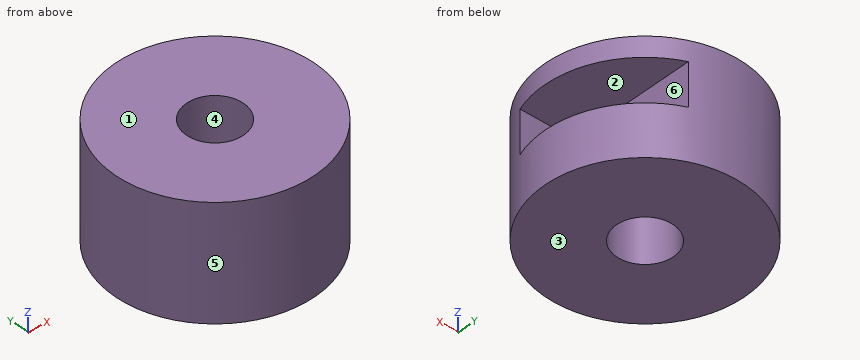
```python
from build123d import *

# Parameters (mm, degrees)
BOX_W             = 30
BOX_H             = 30
BOX_DEPTH         = 7.5
CYLINDER001_R     = 5
CYLINDER001_DEPTH = 40
CYLINDER_R        = 17.5
CYLINDER_DEPTH    = 20


with BuildPart() as cube:
    # Box → Box (new body)
    with BuildSketch(Plane(origin=(7, -6, 9), x_dir=(1, 0, 0), z_dir=(0, 0, 1))):
        with Locations((15, 15)):
            Rectangle(BOX_W, BOX_H)
    extrude(amount=BOX_DEPTH)


with BuildPart() as cylinder001:
    # Cylinder001 → Cylinder001 (new body)
    with BuildSketch(Plane.XY.offset(-10)):
        Circle(CYLINDER001_R)
    extrude(amount=CYLINDER001_DEPTH)


with BuildPart() as mount_bottom:
    # Cylinder → Cylinder (new body)
    with BuildSketch(Plane.XY):
        Circle(CYLINDER_R)
    extrude(amount=CYLINDER_DEPTH)

    # Cut: cut Cylinder001
    add(cylinder001.part, mode=Mode.SUBTRACT)

    # Cut001: cut Cube
    add(cube.part, mode=Mode.SUBTRACT)


solid = mount_bottom.part
```
The listing builds one solid part. Answer for the finished solid, in the listing's coordinates (mm). Face numbers are marked on the shaded views. A direction names the side the tool comes from. Give positions to 0.01 mm unless a question says otherwise; leave off trailing zeros. Order: outer loops, then holes, each group sorted by start corner. A loop starts at its lowest first (then second) coordinate and runs counter-clockwise, first axis right, second up. Notation, with made-up numbers: (80, 32.25) -> (134, 32.25) arc R7 ccw to (134, 44.25) -> close; hole circle Ø11 at (88.5, 77.25). An arc over 180 degrees is marked (long way). One line per item, written item: value.
1) Determine the mould class of the marked faces 3, 4, 5 and 6 for opening direction X: pulls with the +X half, pulls with the -X half, needs draft (parallel to the pull), parting line crosses it, or undercut.
Reported:
face 3: needs draft
face 4: undercut
face 5: parting line crosses it
face 6: pulls with the +X half
2) Find the intervals of material crossed by line 1 (Z direction, x = 15, y = 7); line 2 (Y direction, x = 0, z = 12); line 3 (X direction, y = 3.5, z = 7), in increasing order.
Reported:
line 1: z = 0 to 9, 16.5 to 20
line 2: y = -17.5 to -5, 5 to 17.5
line 3: x = -17.15 to -3.57, 3.57 to 17.15
3) Flat-ended cylindrical pins translate along their axes: P1, Ø1.5, axis at x = -10, z = 13, coming from the -Y side; P2, Ø6, axis at y = 10.5, z = 2.5, coming from the -X side; P3, Ø10, axis at y = 7, z = 7, coming from the +X side; P4, Ø8, axis at y = 3.5, z = 16.5, coming from the +X side. Find the tip coordinate at first contact, or state that the pin passes through.
Reported:
P1: stops at y = -14.86
P2: stops at x = -15.81
P3: stops at x = 17.39
P4: stops at x = 17.5
4) Find section A-A, the plane y = 0. Determine the outline of the cut face in (x, z), plus the area to 3 significant figures.
Reported:
outline: (-17.5, 0) -> (-5, 0) -> (-5, 20) -> (-17.5, 20) -> close; (5, 0) -> (17.5, 0) -> (17.5, 9) -> (7, 9) -> (7, 16.5) -> (17.5, 16.5) -> (17.5, 20) -> (5, 20) -> close
area: 421 mm^2
5) Find section B-B, the plane x = 0. Determine the outline of the cut face in (y, z).
Reported:
outline: (-17.5, 0) -> (-5, 0) -> (-5, 20) -> (-17.5, 20) -> close; (5, 0) -> (17.5, 0) -> (17.5, 20) -> (5, 20) -> close
6) A tool of negligible diameter and unlimited length cuts with its end or side. For the marked faces 1 and 2, from which of +Z, -Z, +X, -X, +Y, -Y can it reach the whole face along a straight path? Write none if from no direction.
Reported:
face 1: +Z, +X, -X, +Y, -Y
face 2: +X, +Y
7) Find section D-D, the plane x = 4.5. Determine the outline of the cut face in (y, z), plus the area to 3 significant figures.
Reported:
outline: (-16.91, 0) -> (-2.18, 0) -> (-2.18, 20) -> (-16.91, 20) -> close; (2.18, 0) -> (16.91, 0) -> (16.91, 20) -> (2.18, 20) -> close
area: 589 mm^2
8) Find section C-C, the plane z = 17. Determine the outline of the cut face in (x, y), plus the area to 3 significant figures.
Reported:
outline: circle Ø35 at (0, 0); hole circle Ø10 at (0, 0)
area: 884 mm^2
